Input: dimensioned drawing with shaded views. Units: mm. Origin: part minimum x, y, z. Give positions to 0.01 mm unless a question says otherwise; leave off trailing zeros. Write each loop counter-clockwise with the first axis right and the second up, starting at its lowest first coordinate (ties: lowest second). Pieces come first, ordered by that corner, then holes.
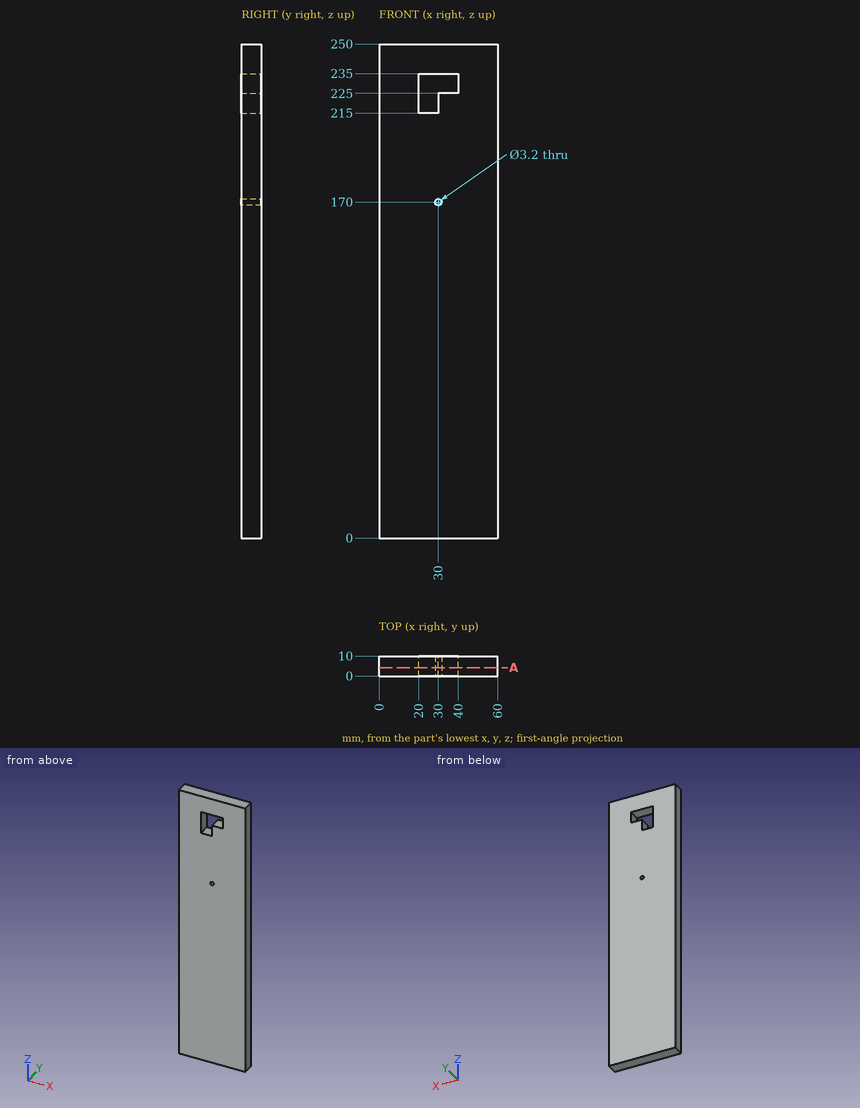
Item 1: Section A-A (y = 4.25). Return loops of the section in (x, z), and give its area (3 significant figures).
Item 2: Pin query (flat end, axial travel): pin 1 (2.5 mm diameter, centred on x = 30, z = 170, fed in from +Y). Return the tip coordinate at first contact, or that it passes through.
Item 3: Ray query, line 1 (X direction, y = 7.5, z = 170); line 2 (Z direction, x = 33, y = 7.25). Return the intervals inside material, ascending.
Solved:
1. outline: (0, 0) - (60, 0) - (60, 250) - (0, 250) - close; hole (20, 215) - (30, 215) - (30, 225) - (40, 225) - (40, 235) - (20, 235) - close; hole circle Ø3.2 at (30, 170)
1. area: 14,700 mm2
2. pin 1: passes through
3. line 1: x = 0 to 28.4, 31.6 to 60
3. line 2: z = 0 to 225, 235 to 250
